The model under review builds one solid part; all positions refer to its coordinate system, in mm. A direction names the side the tool comes from. Give positions to 0.01 mm unless a question says otherwise; leave off trailing zeros.
from build123d import *

# Parameters (mm, degrees)
SKETCH1_R           = 30.25
SKETCH1_R_2         = 25.25
EXTRUDE_THIN1_DEPTH = 1
SKETCH2_R           = 1.65
CUT_EXTRUDE3_DEPTH  = 10
BOSS_EXTRUDE1_DEPTH = 1


with BuildPart() as part:
    # Sketch1 → Extrude-Thin1 (new body)
    with BuildSketch(Plane(origin=(0, 0, 0), x_dir=(1, 0, 0), z_dir=(0, 1, 0))):
        Circle(SKETCH1_R)
        Circle(SKETCH1_R_2, mode=Mode.SUBTRACT)
    extrude(amount=-EXTRUDE_THIN1_DEPTH)

    # Sketch2 → Cut-Extrude3 (cut)
    with BuildSketch(Plane(origin=(0, 0, 0), x_dir=(1, 0, 0), z_dir=(0, 1, 0))):
        with Locations((0, 27.5)):
            Circle(SKETCH2_R)
        with Locations((23.815698604, -13.75)):
            Circle(SKETCH2_R)
        with Locations((-23.815698604, -13.75)):
            Circle(SKETCH2_R)
    extrude(amount=-CUT_EXTRUDE3_DEPTH, mode=Mode.SUBTRACT)

    # Sketch5 → Boss-Extrude1 (add)
    with BuildSketch(Plane.XZ.offset(1)):
        with BuildLine():
            Line((0, 42.25), (0, 30.25))
            ThreePointArc((0, 30.25), (1.319486468, 30.221208703), (2.636461218, 30.134889617))
            Line((2.636461218, 30.134889617), (3.682330131, 42.089225994))
            ThreePointArc((3.682330131, 42.089225994), (1.842919116, 42.209787362), (0, 42.25))
        make_face()
        with BuildLine():
            Line((10.507147733, 40.922638558), (7.522869087, 29.299640624))
            ThreePointArc((7.522869087, 29.299640624), (8.793741356, 28.943610918), (10.047874239, 28.532485403))
            Line((10.047874239, 28.532485403), (14.033807822, 39.851157298))
            ThreePointArc((14.033807822, 39.851157298), (12.28216768, 40.425373926), (10.507147733, 40.922638558))
        make_face()
        with BuildLine():
            Line((20.354092731, 37.023957232), (14.573048642, 26.508277071))
            ThreePointArc((14.573048642, 26.508277071), (15.715453134, 25.847379612), (16.827942369, 25.137280196))
            Line((16.827942369, 25.137280196), (23.503489755, 35.109093827))
            ThreePointArc((23.503489755, 35.109093827), (21.949682477, 36.100885573), (20.354092731, 37.023957232))
        make_face()
        with BuildLine():
            Line((28.922115225, 30.798924509), (20.707549954, 22.051300979))
            ThreePointArc((20.707549954, 22.051300979), (21.649705195, 21.127062384), (22.55064899, 20.162607225))
            Line((22.55064899, 20.162607225), (31.496360987, 28.160996868))
            ThreePointArc((31.496360987, 28.160996868), (30.238017999, 29.508045809), (28.922115225, 30.798924509))
        make_face()
        with BuildLine():
            Line((35.672854852, 22.638682088), (25.540919746, 16.208760548))
            ThreePointArc((25.540919746, 16.208760548), (26.223626655, 15.079254128), (26.8564154, 13.92104349))
            Line((26.8564154, 13.92104349), (37.510200022, 19.443440907))
            ThreePointArc((37.510200022, 19.443440907), (36.626387643, 21.061107005), (35.672854852, 22.638682088))
        make_face()
        with BuildLine():
            Line((40.182137813, 13.055968012), (28.769459618, 9.34776408))
            ThreePointArc((28.769459618, 9.34776408), (29.14982121, 8.083960876), (29.47469446, 6.804769394))
            Line((29.47469446, 6.804769394), (41.167135237, 9.504182046))
            ThreePointArc((41.167135237, 9.504182046), (40.713386648, 11.290821389), (40.182137813, 13.055968012))
        make_face()
        with BuildLine():
            Line((42.166629276, 2.65289945), (30.190308535, 1.899413216))
            ThreePointArc((30.190308535, 1.899413216), (30.244425292, 0.580722633), (30.240970066, -0.739073389))
            Line((30.240970066, -0.739073389), (42.237387943, -1.032259527))
            ThreePointArc((42.237387943, -1.032259527), (42.242213837, 0.811091941), (42.166629276, 2.65289945))
        make_face()
        with BuildLine():
            Line((41.501636343, -7.916860541), (29.714189335, -5.668284766))
            ThreePointArc((29.714189335, -5.668284766), (29.438660902, -6.95900455), (29.107094304, -8.236477473))
            Line((29.107094304, -8.236477473), (40.653710227, -11.503840437))
            ThreePointArc((40.653710227, -11.503840437), (41.116807375, -9.719601396), (41.501636343, -7.916860541))
        make_face()
        with BuildLine():
            Line((38.228942967, -17.989175069), (27.371018337, -12.87982357))
            ThreePointArc((27.371018337, -12.87982357), (26.783157179, -14.061471883), (26.144312759, -15.216353386))
            Line((26.144312759, -15.216353386), (36.515610383, -21.252592745))
            ThreePointArc((36.515610383, -21.252592745), (37.407880688, -19.639576432), (38.228942967, -17.989175069))
        make_face()
        with BuildLine():
            Line((32.554184507, -26.931163567), (23.308025594, -19.28207569))
            ThreePointArc((23.308025594, -19.28207569), (22.44476919, -20.280405224), (21.538787891, -21.240129853))
            Line((21.538787891, -21.240129853), (30.083100443, -29.665966489))
            ThreePointArc((30.083100443, -29.665966489), (31.348479281, -28.325524651), (32.554184507, -26.931163567))
        make_face()
        with BuildLine():
            Line((24.833926909, -34.180968012), (17.780503882, -24.47276408))
            ThreePointArc((17.780503882, -24.47276408), (16.696093806, -25.225046118), (15.579901766, -25.929310846))
            Line((15.579901766, -25.929310846), (21.760358665, -36.215318455))
            ThreePointArc((21.760358665, -36.215318455), (23.319337629, -35.231675982), (24.833926909, -34.180968012))
        make_face()
        with BuildLine():
            Line((15.553262351, -39.283056529), (11.135767719, -28.125738698))
            ThreePointArc((11.135767719, -28.125738698), (9.898341444, -28.584704593), (8.642073114, -28.989257878))
            Line((8.642073114, -28.989257878), (12.070333523, -40.489128771))
            ThreePointArc((12.070333523, -40.489128771), (13.824956232, -39.924091539), (15.553262351, -39.283056529))
        make_face()
        with BuildLine():
            Line((5.295329118, -41.916846131), (3.791330315, -30.011469715))
            ThreePointArc((3.791330315, -30.011469715), (2.478639886, -30.148280951), (1.161231225, -30.227703221))
            Line((1.161231225, -30.227703221), (1.621884934, -42.218858218))
            ThreePointArc((1.621884934, -42.218858218), (3.46190199, -42.107929593), (5.295329118, -41.916846131))
        make_face()
        with BuildLine():
            Line((-5.295329118, -41.916846131), (-3.791330315, -30.011469715))
            ThreePointArc((-3.791330315, -30.011469715), (-5.096803732, -29.81752994), (-6.392575093, -29.566830802))
            Line((-6.392575093, -29.566830802), (-8.92847265, -41.295821534))
            ThreePointArc((-8.92847265, -41.295821534), (-7.118676287, -41.645971569), (-5.295329118, -41.916846131))
        make_face()
        with BuildLine():
            Line((-15.553262351, -39.283056529), (-11.135767719, -28.125738698))
            ThreePointArc((-11.135767719, -28.125738698), (-12.351996427, -27.613233861), (-13.544712407, -27.048165664))
            Line((-13.544712407, -27.048165664), (-18.917821461, -37.778016506))
            ThreePointArc((-18.917821461, -37.778016506), (-17.251961951, -38.567243988), (-15.553262351, -39.283056529))
        make_face()
        with BuildLine():
            Line((-24.833926909, -34.180968012), (-17.780503882, -24.47276408))
            ThreePointArc((-17.780503882, -24.47276408), (-18.831067758, -23.673896745), (-19.845785627, -22.829964802))
            Line((-19.845785627, -22.829964802), (-27.718493975, -31.886479764))
            ThreePointArc((-27.718493975, -31.886479764), (-26.301243398, -33.065194627), (-24.833926909, -34.180968012))
        make_face()
        with BuildLine():
            Line((-32.554184507, -26.931163567), (-23.308025594, -19.28207569))
            ThreePointArc((-23.308025594, -19.28207569), (-24.126913847, -18.247041629), (-24.899875148, -17.177273288))
            Line((-24.899875148, -17.177273288), (-34.777511571, -23.991398228))
            ThreePointArc((-34.777511571, -23.991398228), (-33.697920993, -25.485537482), (-32.554184507, -26.931163567))
        make_face()
        with BuildLine():
            Line((-38.228942967, -17.989175069), (-27.371018337, -12.87982357))
            ThreePointArc((-27.371018337, -12.87982357), (-27.906777206, -11.67365778), (-28.389413938, -10.44527052))
            Line((-28.389413938, -10.44527052), (-39.651330212, -14.588848908))
            ThreePointArc((-39.651330212, -14.588848908), (-38.97723428, -16.304530288), (-38.228942967, -17.989175069))
        make_face()
        with BuildLine():
            Line((-41.501636343, -7.916860541), (-29.714189335, -5.668284766))
            ThreePointArc((-29.714189335, -5.668284766), (-29.933155119, -4.36677508), (-30.095141442, -3.05695299))
            Line((-30.095141442, -3.05695299), (-42.033709948, -4.269628556))
            ThreePointArc((-42.033709948, -4.269628556), (-41.807464588, -6.099049492), (-41.501636343, -7.916860541))
        make_face()
        with BuildLine():
            Line((-42.166629276, 2.65289945), (-30.190308535, 1.899413216))
            ThreePointArc((-30.190308535, 1.899413216), (-30.07872281, 3.214488158), (-29.909880527, 4.523444139))
            Line((-29.909880527, 4.523444139), (-41.774957099, 6.31786826))
            ThreePointArc((-41.774957099, 6.31786826), (-42.01077814, 4.489657014), (-42.166629276, 2.65289945))
        make_face()
        with BuildLine():
            Line((-40.182137813, 13.055968012), (-28.769459618, 9.34776408))
            ThreePointArc((-28.769459618, 9.34776408), (-28.334333725, 10.593773283), (-27.845271817, 11.819616637))
            Line((-27.845271817, 11.819616637), (-38.891330058, 16.508390179))
            ThreePointArc((-38.891330058, 16.508390179), (-39.574399996, 14.796261858), (-40.182137813, 13.055968012))
        make_face()
        with BuildLine():
            Line((-35.672854852, 22.638682088), (-25.540919746, 16.208760548))
            ThreePointArc((-25.540919746, 16.208760548), (-24.809594245, 17.307412672), (-24.031042271, 18.373119152))
            Line((-24.031042271, 18.373119152), (-33.564017718, 25.661629228))
            ThreePointArc((-33.564017718, 25.661629228), (-34.651416756, 24.173163153), (-35.672854852, 22.638682088))
        make_face()
        with BuildLine():
            Line((-28.922115225, 30.798924509), (-20.707549954, 22.051300979))
            ThreePointArc((-20.707549954, 22.051300979), (-19.725976716, 22.93356367), (-18.70685396, 23.772171019))
            Line((-18.70685396, 23.772171019), (-26.127754704, 33.202453737))
            ThreePointArc((-26.127754704, 33.202453737), (-27.551157562, 32.031175704), (-28.922115225, 30.798924509))
        make_face()
        with BuildLine():
            Line((-20.354092731, 37.023957232), (-14.573048642, 26.508277071))
            ThreePointArc((-14.573048642, 26.508277071), (-13.402903522, 27.118714519), (-12.207245215, 27.677529952))
            Line((-12.207245215, 27.677529952), (-17.049788771, 38.657045967))
            ThreePointArc((-17.049788771, 38.657045967), (-18.719757812, 37.876551684), (-20.354092731, 37.023957232))
        make_face()
        with BuildLine():
            Line((-10.507147733, 40.922638558), (-7.522869087, 29.299640624))
            ThreePointArc((-7.522869087, 29.299640624), (-6.237676608, 29.599896799), (-4.940610358, 29.843807889))
            Line((-4.940610358, 29.843807889), (-6.900521905, 41.682673828))
            ThreePointArc((-6.900521905, 41.682673828), (-8.712126833, 41.342004621), (-10.507147733, 40.922638558))
        make_face()
    extrude(amount=-BOSS_EXTRUDE1_DEPTH)


solid = part.part
1) The part is to be moulded in two halves that separate along X. For faces 5 (the flat face through (-33.942, -0.507, -12.488)), 6 (the cylindrical face through (13.434, -0.493, -27.103)), 7 (the cylindrical face through (30.256, -0.507, 29.49)), say which applies: +X half, -X half, draft (parallel to the pull), parting line (faces both ways), or undercut.
2) To check wall thickness, follow probe 1 along X at (y, z) = (-0.05, -28); probe 2 along Z at (x, y) = (20.5, -0.15); probe 3 along X at (y, z) = (-0.3, 20.5). State the ranges of each line that lie inside material, in increasing order.
3) Tool access review of faces 1 (the cylindrical face through (-27.53, -0.51, 32.05)), 2 (the flat face through (18.627, -0.507, -31)), 3 (the flat face through (-14.6, -0.5, 33.1)), 4 (the flat face through (20.119, -0.507, 30.053)): name each direction out of +Z, -Z, +X, -X, +Y, -Y from which nothing blocks a thin tool from reaching the whole face with its end or side.
4) Consider section A-A, the plane y = -0.55. State how many separate pieces and enclosed holes the cut face has, then the cut area to 3 significant figures.
Answer block:
1. face 5: -X half
1. face 6: undercut
1. face 7: +X half
2. probe 1: x = -24.34 to -20.34, -14.02 to -1.57, 1.57 to 11.45, 16.82 to 20.34, 28.39 to 31.64
2. probe 2: z = -34.12 to -28.22, -22.24 to -14.74, 14.74 to 22.24, 30.62 to 36.94
2. probe 3: x = -32.3 to -26.81, -22.24 to -14.74, 14.74 to 22.93, 32.3 to 36.94
3. face 1: +Z, -X, +Y, -Y
3. face 2: -Z, +Y, -Y
3. face 3: +Z, +Y, -Y
3. face 4: +Y, -Y
4. separate pieces: 1
4. enclosed holes: 4
4. area: 1,800 mm2
